Verification items for the finished model (mm, model axes). Give positions to 0.01 mm unless a question says otherwise; leave off trailing zeros. Order: outer loops, then holes, each group sorted by start corner. A loop starts at its lowest first (then second) coordinate and runs counter-clockwise, first axis right, second up.
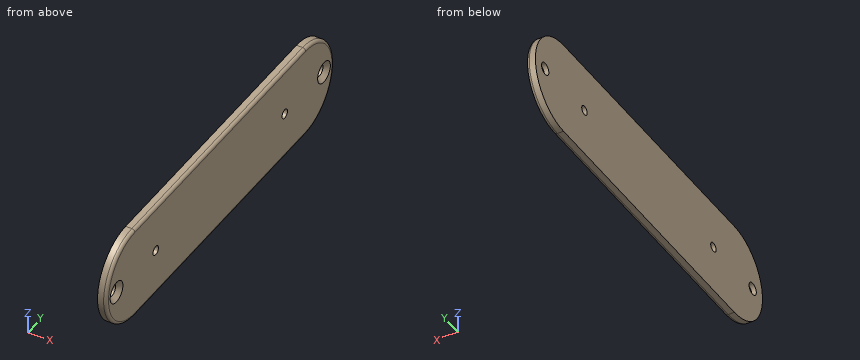
from build123d import *

# Parameters (mm, degrees)
F0_R     = 2
F0_R_2   = 1.5
F1_DEPTH = 1.5
F2_SIZE  = 1.5
F3_R     = 1


with BuildPart() as f1:
    # F0 (on Right) → F1 (new body, symmetric)
    with BuildSketch(Plane.YZ):
        with BuildLine():
            Line((47, 15.5), (0, 15.5))
            Line((0, 15.5), (-47, 15.5))
            ThreePointArc((-47, 15.5), (-62.5, 0), (-47, -15.5))
            Line((-47, -15.5), (0, -15.5))
            Line((0, -15.5), (47, -15.5))
            ThreePointArc((47, -15.5), (62.5, 0), (47, 15.5))
        make_face()
        with Locations((-57.09, 0)):
            Circle(F0_R, mode=Mode.SUBTRACT)
        with Locations((-35.5, 0)):
            Circle(F0_R_2, mode=Mode.SUBTRACT)
        with Locations((35.5, 0)):
            Circle(F0_R_2, mode=Mode.SUBTRACT)
        with Locations((57.09, 0)):
            Circle(F0_R, mode=Mode.SUBTRACT)
    extrude(amount=F1_DEPTH, both=True)

    # F2
    f2_edges = [f1.edges().sort_by_distance(p)[0] for p in [
        (1.5, -59.09, 0),
        (1.5, 55.09, 0),
    ]]
    chamfer(f2_edges, length=F2_SIZE)

    # F3
    f3_edges = [f1.edges().sort_by_distance(p)[0] for p in [
        (1.5, 0, -15.5),
    ]]
    fillet(f3_edges, radius=F3_R)


solid = f1.part
(1) Section check B-B, the plane x = -1. Enter the section's corners in (y, z), then the cut area to 3 significant figures.
Solved:
outline: (-47, -15.5) - (47, -15.5) arc R15.5 ccw to (47, 15.5) - (-47, 15.5) arc R15.5 ccw to start; hole circle Ø4 at (-57.09, 0); hole circle Ø3 at (-35.5, 0); hole circle Ø3 at (35.5, 0); hole circle Ø4 at (57.09, 0)
area: 3,630 mm2
(2) Section check C-C, the plane z = 0. Enter the section's corners in (x, y).
Solved:
outline: (-1.5, -62.5) - (0.5, -62.5) arc R1 ccw to (1.5, -61.5) - (1.5, -60.59) - (0, -59.09) - (-1.5, -59.09) - close; (-1.5, -55.09) - (0, -55.09) - (1.5, -53.59) - (1.5, -37) - (-1.5, -37) - close; (-1.5, -34) - (1.5, -34) - (1.5, 34) - (-1.5, 34) - close; (-1.5, 37) - (1.5, 37) - (1.5, 53.59) - (0, 55.09) - (-1.5, 55.09) - close; (-1.5, 59.09) - (0, 59.09) - (1.5, 60.59) - (1.5, 61.5) arc R1 ccw to (0.5, 62.5) - (-1.5, 62.5) - close
(3) Scan lines: line 1 (Z direction, x = -0.75, y = 56); line 2 (Z direction, x = -0.8, y = -57.09); line 3 (Y direction, x = -1.1, z = 3). Record each from-to range of solid material in increasing order.
Solved:
line 1: z = -12.62 to -1.68, 1.68 to 12.62
line 2: z = -11.77 to -2, 2 to 11.77
line 3: y = -62.21 to 62.21
(4) Section check A-A, the plane y = 35.5. Enter the section's corners in (x, z), then the cut area to 3 significant figures.
Solved:
outline: (-1.5, -15.5) - (0.5, -15.5) arc R1 ccw to (1.5, -14.5) - (1.5, -1.5) - (-1.5, -1.5) - close; (-1.5, 1.5) - (1.5, 1.5) - (1.5, 14.5) arc R1 ccw to (0.5, 15.5) - (-1.5, 15.5) - close
area: 83.6 mm2
(5) Go/stop test with flat-tipped pins: pin 1 (1.8 mm diameter, centred on y = -35.5, z = 0, fed in from -X) (3 decimals); pin 2 (5 mm diameter, centred on y = -57.09, z = 0, fed in from +X). Record where each tip stops, or that it passes through.
Solved:
pin 1: passes through
pin 2: stops at x = 0.5
